Here's how the part is built. I have some questions about the finished solid (model axes, mm). Face numbers are marked on the shaded views. Coordinates: 2 decimals unless noted, no trailing zeros. Write each loop counter-clockwise with the first axis right and the second up, starting at its lowest first coordinate (ties: lowest second). Pieces come first, ordered by that corner, then holes. Notation, with made-up numbers: (-10.75, -13.5) -> (5.25, -13.5) arc R18 cw to (5.25, 0.5) -> close; hole circle Ø7 at (-37.75, -35). An arc over 180 degrees is marked (long way). Put each result on its own line as item: value.
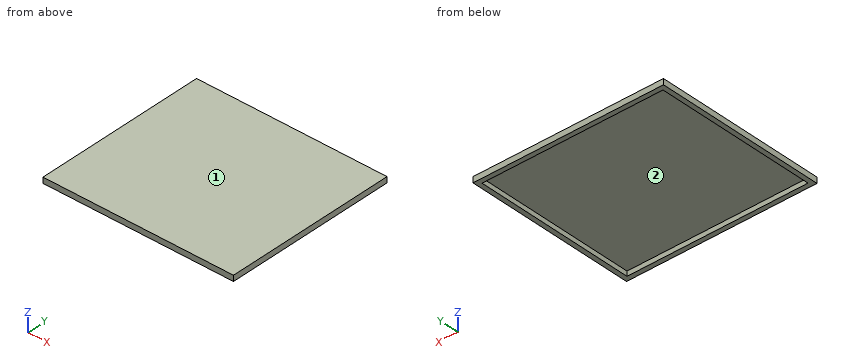
```python
from build123d import *

# Parameters (mm, degrees)
F0_W     = 1000
F0_H     = 900
F1_DEPTH = 30
F2_W     = 950
F2_H     = 850
F3_DEPTH = 25


with BuildPart() as f1:
    # F0 (on Top) → F1 (new body)
    with BuildSketch(Plane.XY):
        Rectangle(F0_W, F0_H)
    extrude(amount=F1_DEPTH)

    # F2 (on face) → F3 (cut)
    with BuildSketch(Plane(origin=(0, 0, 0), x_dir=(1, 0, 0), z_dir=(0, 0, -1))):
        Rectangle(F2_W, F2_H)
    extrude(amount=-F3_DEPTH, mode=Mode.SUBTRACT)


solid = f1.part
```
Item 1: Imagine slicing it at A-A on z = 10. Write out the boundary of the cut face in (x, y).
Output:
outline: (-500, -450) -> (500, -450) -> (500, 450) -> (-500, 450) -> close; hole (-475, -425) -> (475, -425) -> (475, 425) -> (-475, 425) -> close
Item 2: Please list where these lines run through material, in increasing order: line 1 along Y through (x, z) = (-50, 9.75); line 2 along X through (y, z) = (-363.5, 1.75); line 3 along Z through (x, y) = (-352.5, 150). Write a range as from..to.
Output:
line 1: y = -450..-425, 425..450
line 2: x = -500..-475, 475..500
line 3: z = 25..30
Item 3: If we mould it in two halves opening along X, with no side actions, what happens to the marked faces 1 and 2? For each: released by +X, released by -X, zero draft, split by the parting line, or undercut.
Output:
face 1: zero draft
face 2: undercut
Item 4: Imagine slicing it at C-C on x = -256. Write out the boundary of the cut face in (y, z).
Output:
outline: (-450, 0) -> (-425, 0) -> (-425, 25) -> (425, 25) -> (425, 0) -> (450, 0) -> (450, 30) -> (-450, 30) -> close
Item 5: Imagine slicing it at B-B on y = -25.5. Write out the boundary of the cut face in (x, z), then the cut area to 3 significant figures.
Output:
outline: (-500, 0) -> (-475, 0) -> (-475, 25) -> (475, 25) -> (475, 0) -> (500, 0) -> (500, 30) -> (-500, 30) -> close
area: 6,250 mm²
